from build123d import *

# Parameters (mm, degrees)
SKETCH1_W           = 72
SKETCH1_H           = 58.3
SKETCH1_R           = 10
SKETCH1_R_2         = 1.45
SKETCH1_R_3         = 1.3
BOSS_EXTRUDE1_DEPTH = 5
SKETCH2_W           = 46.5
SKETCH2_H           = 52
SKETCH2_R           = 1.45
BOSS_EXTRUDE2_DEPTH = 5.5
SKETCH3_R           = 7.6
CUT_EXTRUDE1_DEPTH  = 1.2
SKETCH4_W           = 46.5
SKETCH4_H           = 52
SKETCH4_R           = 2.6
BOSS_EXTRUDE3_DEPTH = 5.5
CUT_EXTRUDE2_DEPTH  = 3.6


with BuildPart() as part:
    # Sketch1 → Boss-Extrude1 (new body)
    with BuildSketch(Plane.XY.offset(280)):
        with Locations((300, 299.15)):
            Rectangle(SKETCH1_W, SKETCH1_H)
        with Locations((300, 300)):
            Circle(SKETCH1_R, mode=Mode.SUBTRACT)
        with Locations((286.774831823, 318.202882373)):
            Circle(SKETCH1_R_2, mode=Mode.SUBTRACT)
        with Locations((278.601228383, 293.047117627)):
            Circle(SKETCH1_R_2, mode=Mode.SUBTRACT)
        with Locations((300, 277.5)):
            Circle(SKETCH1_R_2, mode=Mode.SUBTRACT)
        with Locations((321.398771617, 293.047117627)):
            Circle(SKETCH1_R_2, mode=Mode.SUBTRACT)
        with Locations((313.225168177, 318.202882373)):
            Circle(SKETCH1_R_2, mode=Mode.SUBTRACT)
        with Locations((295, 324)):
            Circle(SKETCH1_R_3, mode=Mode.SUBTRACT)
        with Locations((305, 324)):
            Circle(SKETCH1_R_3, mode=Mode.SUBTRACT)
    extrude(amount=BOSS_EXTRUDE1_DEPTH)

    # Sketch2 → Boss-Extrude2 (add)
    with BuildSketch(Plane(origin=(264, 0, 0), x_dir=(0, 0, -1), z_dir=(1, 0, 0))):
        with Locations((-303.25, 300)):
            Rectangle(SKETCH2_W, SKETCH2_H)
        with Locations((-300, 313.5)):
            Circle(SKETCH2_R, mode=Mode.SUBTRACT)
        with Locations((-288.308657049, 293.25)):
            Circle(SKETCH2_R, mode=Mode.SUBTRACT)
        with Locations((-311.691342951, 293.25)):
            Circle(SKETCH2_R, mode=Mode.SUBTRACT)
    extrude(amount=BOSS_EXTRUDE2_DEPTH)

    # Sketch3 → Cut-Extrude1 (cut)
    with BuildSketch(Plane(origin=(264, 0, 0), x_dir=(0, 0, -1), z_dir=(1, 0, 0))):
        with Locations((-300, 300)):
            Circle(SKETCH3_R)
    extrude(amount=CUT_EXTRUDE1_DEPTH, mode=Mode.SUBTRACT)

    # Sketch4 → Boss-Extrude3 (add)
    with BuildSketch(Plane(origin=(330.5, 0, 0), x_dir=(0, 0, -1), z_dir=(1, 0, 0))):
        with Locations((-303.25, 300)):
            Rectangle(SKETCH4_W, SKETCH4_H)
        with Locations((-300, 300)):
            Circle(SKETCH4_R, mode=Mode.SUBTRACT)
    extrude(amount=BOSS_EXTRUDE3_DEPTH)

    # Sketch5 → Cut-Extrude2 (cut)
    with BuildSketch(Plane(origin=(330.5, 0, 0), x_dir=(0, 0, -1), z_dir=(1, 0, 0))):
        Polygon((-304.1, 302.367136104), (-300, 304.734272207), (-295.9, 302.367136104), (-295.9, 297.632863896), (-300, 295.265727793), (-304.1, 297.632863896), align=None)
    extrude(amount=CUT_EXTRUDE2_DEPTH, mode=Mode.SUBTRACT)


solid = part.part
Model file for the job. Use its own axes, mm. A direction names the side the tool comes from. Give positions to 0.01 mm unless a question says otherwise; leave off trailing zeros. Write each loop counter-clockwise with the first axis right and the second up, starting at its lowest first coordinate (ties: lowest second). Pieces come first, ordered by that corner, then holes. Notation, with made-up numbers: M 74.25,-29 L 127.25,-29 A12 cw 127.25,-20 Z; hole C -33,-21.5 d6. An arc over 180 degrees is marked long. One line per item, written item: value. Start each with the question number.
Q1. Probe probe 1 along X at (y, z) = (324, 283.6); probe 2 along X at (y, z) = (285.5, 294); probe 3 along X at (y, z) = (298, 298). List the from-to ranges inside material, lowest first. Write a range as [from, to].
Q2. Drop flat-ended pins along their axis: pin 1 Ø7.5 at (y, z) = (302, 299.5) entering from -X; pin 2 Ø8 at (x, y) = (292, 291) entering from +Z; pin 3 Ø2.5 at (x, y) = (295, 324) entering from +Z; pin 4 Ø1.7 at (y, z) = (293.25, 288.31) entering from -X. Give the stop position or say it passes through.
Q3. Saw through at B-B, the plane y = 300. Write the cut outline in (x, z).
Q4. 3-axis set-ups, long thin cutter, end or side, ignore diameter. For faces 4 (the flat face through (267, 326, 306)), 5 (the flat face through (267, 274, 306)), 6 (the flat face through (332, 300, 295.9)), 7 (the cylindrical face through (264.59, 292.58, 301.65)): which of +Z, -Z, +X, -X, +Y, -Y reach the whole face in a straight line?
Q5. Saw through at A-A, the plane y = 277.5. Write the cut outline in (x, z), plus the area to 3 significant figures.
Q6. Saw through at C-C, the plane z = 315.5. Write the cut outline in (x, y), plus the area to 3 significant figures.
Q7. Saw through at D-D, the plane x = 305. Write the cut outline in (y, z).
Q8. Two-plate mould, pull along X, no slides. Class faces 1 (the flat face through (265.2, 300, 300)), 2 (the cylindrical face through (293.97, 323.21, 282.46)), 3 (the flat face through (291, 292, 280)): +X half, -X half, draft (parallel to the pull), parting line (faces both ways), or undercut.
Output values:
1. probe 1: x = [264, 293.7], [296.3, 303.7], [306.3, 336]
1. probe 2: x = [264, 269.5], [330.5, 336]
1. probe 3: x = [265.2, 269.5], [334.1, 336]
2. pin 1: stops at x = 265.2
2. pin 2: stops at z = 285
2. pin 3: passes through
2. pin 4: stops at x = 330.5
3. outline: M 264,280 L 290,280 L 290,285 L 269.5,285 L 269.5,326.5 L 264,326.5 L 264,307.6 L 265.2,307.6 L 265.2,292.4 L 264,292.4 Z; M 310,280 L 336,280 L 336,297.4 L 334.1,297.4 L 334.1,295.9 L 330.5,295.9 L 330.5,285 L 310,285 Z; M 330.5,304.1 L 334.1,304.1 L 334.1,302.6 L 336,302.6 L 336,326.5 L 330.5,326.5 Z
4. face 4: +Z, +X, -X, +Y
4. face 5: +Z, +X, -X, -Y
4. face 6: none
4. face 7: -X
5. outline: M 264,280 L 298.55,280 L 298.55,285 L 269.5,285 L 269.5,326.5 L 264,326.5 Z; M 301.45,280 L 336,280 L 336,326.5 L 330.5,326.5 L 330.5,285 L 301.45,285 Z
5. area: 802 mm²
6. outline: M 264,274 L 269.5,274 L 269.5,326 L 264,326 Z; M 330.5,274 L 336,274 L 336,326 L 330.5,326 Z
6. area: 572 mm²
7. outline: M 270,280 L 291.34,280 L 291.34,285 L 270,285 Z; M 308.66,280 L 322.7,280 L 322.7,285 L 308.66,285 Z; M 325.3,280 L 328.3,280 L 328.3,285 L 325.3,285 Z
8. face 1: -X half
8. face 2: undercut
8. face 3: draft
